```python
from build123d import *

# Parameters (mm, degrees)
SKETCH_1_W          = 48
SKETCH_1_H          = 10
SKETCH_1_R          = 2
EXTRUDE_1_DEPTH     = 10
SKETCH_2_R          = 2
CUT_EXTRUDE_1_DEPTH = 10


with BuildPart() as part:
    # 草图1 → 凸台-拉伸1 (new body)
    with BuildSketch(Plane(origin=(0, 0, 0), x_dir=(1, 0, 0), z_dir=(0, 1, 0))):
        Rectangle(SKETCH_1_W, SKETCH_1_H)
        with Locations(Location((16, 0, 0), (0, 0, 270))):
            Circle(SKETCH_1_R, mode=Mode.SUBTRACT)
        with Locations(Location((-16, 0, 0), (0, 0, 270))):
            Circle(SKETCH_1_R, mode=Mode.SUBTRACT)
    extrude(amount=EXTRUDE_1_DEPTH)

    # 草图2 → 切除-拉伸1 (cut)
    with BuildSketch(Plane.XY.offset(5)):
        with Locations((-8, 5)):
            Circle(SKETCH_2_R)
        with Locations((8, 5)):
            Circle(SKETCH_2_R)
    extrude(amount=-CUT_EXTRUDE_1_DEPTH, mode=Mode.SUBTRACT)


solid = part.part
```
The model under review builds one solid part; all positions refer to its coordinate system, in mm. Round coordinates to 2 decimals unless told otherwise and drop trailing zeros. Write each loop counter-clockwise with the first axis right and the second up, starting at its lowest first coordinate (ties: lowest second). Pieces come first, ordered by that corner, then holes. Notation, with made-up numbers: (28.5, -28) - (64.5, -28) arc R26 cw to (64.5, 3) - close; hole circle Ø5 at (39, 16.25). An arc over 180 degrees is marked (long way). Answer as CSV lines item,"result". Start each with the question number.
(1) We need section C-C on z = 0. State the section outline as (x, y) points.
(2) For pin 1 Ø3.5 at (x, y) = (-8, 5) entering from +Z, flat-tipped, find the tip position at first contact; note if it passes through.
(3) We need section A-A on y = 5. State the section outline as (x, z) points, plus the area to 3 significant figures.
(4) To check wall thickness, follow line 1 (X direction, y = 7.75, z = 0); line 2 (Y direction, x = 8, z = -1.25); line 3 (X direction, y = 3.75, z = 0). State the ranges of each line that lie inside material, in increasing order.
(5) We need section D-D on y = 9.25. State the section outline as (x, z) points.
(6) We need section B-B on x = 16. State the section outline as (y, z) points.
(7) Draft analysis for pull direction Y (two halves, no side actions). For faces 1 (the cylindrical face through (-10, 5, 0)), 2 (the flat face through (0, 5, 5)), 3 (the flat face through (0, 10, 0)), state which applies: pulls with the +Y half, pulls with the -Y half, needs draft (parallel to the pull), parting line crosses it, or undercut.
Worked answers:
1,outline,"(-24, 0) - (-18, 0) - (-18, 10) - (-24, 10) - close; (-14, 0) - (14, 0) - (14, 10) - (-14, 10) - close; (18, 0) - (24, 0) - (24, 10) - (18, 10) - close; hole circle Ø4 at (-8, 5); hole circle Ø4 at (8, 5)"
2,pin 1,"through"
3,outline,"(-24, -5) - (-10, -5) - (-10, 5) - (-24, 5) - close; (-6, -5) - (6, -5) - (6, 5) - (-6, 5) - close; (10, -5) - (24, -5) - (24, 5) - (10, 5) - close; hole circle Ø4 at (-16, 0); hole circle Ø4 at (16, 0)"
3,area,"375 mm²"
4,line 1,"-24 to -18, -14 to 14, 18 to 24"
4,line 2,"0 to 3, 7 to 10"
4,line 3,"-24 to -18, -14 to -9.56, -6.44 to 6.44, 9.56 to 14, 18 to 24"
5,outline,"(-24, -5) - (24, -5) - (24, 5) - (-24, 5) - close; hole circle Ø4 at (-16, 0); hole circle Ø4 at (16, 0)"
6,outline,"(0, -5) - (10, -5) - (10, -2) - (0, -2) - close; (0, 2) - (10, 2) - (10, 5) - (0, 5) - close"
7,face 1,"undercut"
7,face 2,"needs draft"
7,face 3,"pulls with the +Y half"
